Could you check a few things on this drawing? It's one solid part, dimensions in mm from its lowest x, y, z. A direction names the side the tool comes from. Give positions to 0.01 mm unless a question says otherwise; leave off trailing zeros. Order: outer loops, then holes, each group sorted by start corner. A loop starts at its lowest first (then second) coordinate and runs counter-clockwise, first axis right, second up. Notation, with made-up numbers: (88.25, 10) - (144.25, 10) arc R16 cw to (144.25, 16) - close; hole circle Ø10 at (21.25, 22). An arc over 180 degrees is marked (long way). Answer as CSV lines item,"result".
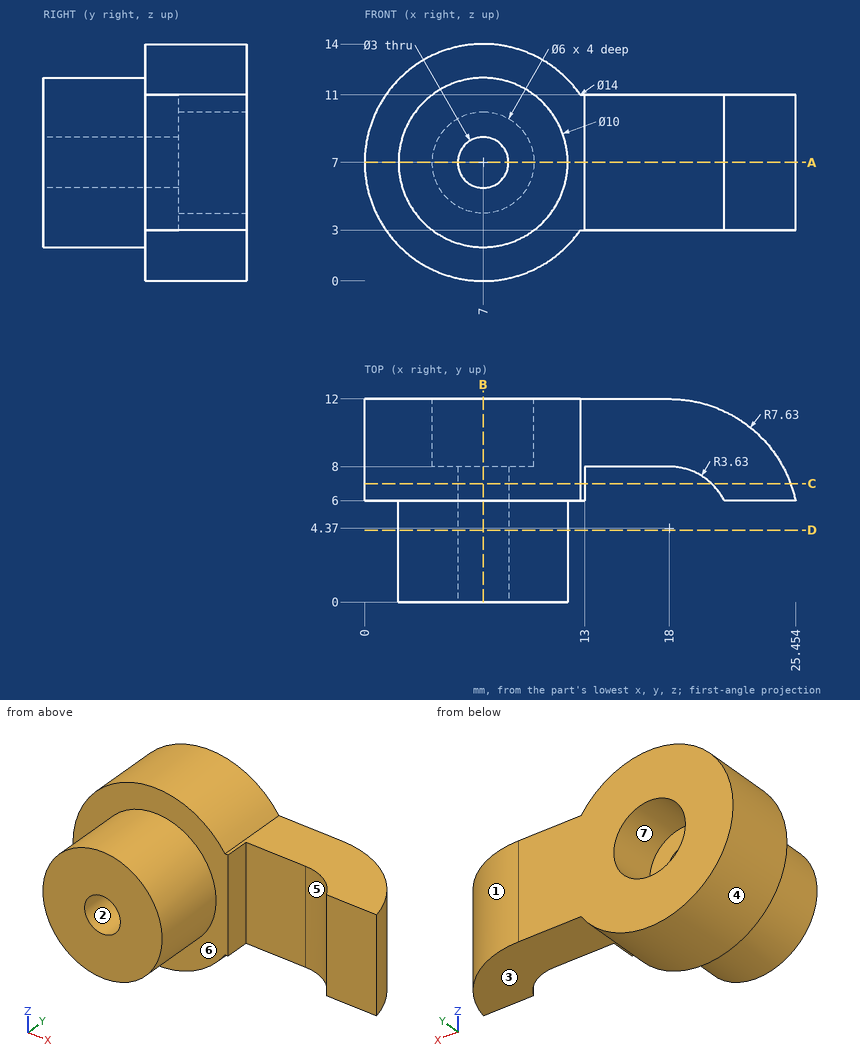
1) I want a section at D-D on y = 4.25. Write out the boundary of the cut face in (x, z).
Answer block:
outline,"circle Ø10 at (7, 7); hole circle Ø3 at (7, 7)"
2) I want a section at B-B on x = 7. Write out the boundary of the cut face in (y, z), plus the area to 3 significant figures.
Answer block:
outline,"(0, 2) - (6, 2) - (6, 0) - (12, 0) - (12, 4) - (8, 4) - (8, 5.5) - (0, 5.5) - close; (0, 8.5) - (8, 8.5) - (8, 10) - (12, 10) - (12, 14) - (6, 14) - (6, 12) - (0, 12) - close"
area,"96.0 mm2"
3) I need wall thicknesses on line 1 along Y through (x, z) = (15.25, 8); line 2 along Z through (x, y) = (5.75, 7.5); line 3 along X through (y, z) = (10.25, 7). Which ranges of each line are inside material? Lowest first, please. Write a range as [from, to].
Answer block:
line 1,"[8, 12]"
line 2,"[0.11, 6.17], [7.83, 13.89]"
line 3,"[0, 4], [10, 22.86]"
4) If we mould it in two halves opening along Z, with no side actions, what happens to the marked faces 1, 2, 3 and 4? For each: +Z half, -Z half, draft (parallel to the pull), parting line (faces both ways), or undercut.
Answer block:
face 1,"draft"
face 2,"undercut"
face 3,"-Z half"
face 4,"parting line"
5) I want a section at A-A on z = 7. Write out the boundary of the cut face in (x, y), plus the area to 3 significant figures.
Answer block:
outline,"(0, 6) - (2, 6) - (2, 0) - (5.5, 0) - (5.5, 8) - (4, 8) - (4, 12) - (0, 12) - close; (8.5, 0) - (12, 0) - (12, 6) - (13, 6) - (13, 8) - (18, 8) arc R3.63 cw to (21.24, 6) - (25.45, 6) arc R7.63 ccw to (18, 12) - (10, 12) - (10, 8) - (8.5, 8) - close"
area,"139 mm2"
6) Which directions (+Z, -Z, +X, -X, +Y, -Y) give clear straight access to the entire face, cutting with the end or side of a thin tool? Please do the marked faces 5, 6 and 7.
Answer block:
face 5,"+Z, -Z, -Y"
face 6,"-Y"
face 7,"+Y"
7) I want a section at C-C on y = 7. Write out the boundary of the cut face in (x, z), plus the area to 3 significant figures.
Answer block:
outline,"(12.74, 3) - (13, 3) - (13, 11) - (12.74, 11) arc R7 ccw (long way) to start; (20.5, 3) - (25.16, 3) - (25.16, 11) - (20.5, 11) - close; hole circle Ø3 at (7, 7)"
area,"179 mm2"
8) I'm going to push flat-ended pins straight in: P1, Ø5, axis at x = 19, y = 10, coming from the -Z side; P2, Ø2, axis at x = 16.5, z = 7, coming from the -Y side; P3, Ø1.3, axis at x = 23.5, z = 5, coming from the -Y side; P4, Ø4, axis at x = 21, y = 3, coming from the +Z side. Where does each tip first touch, or does it pass through?
Answer block:
P1,"z = 3"
P2,"y = 8"
P3,"y = 6"
P4,"through"
